For this review, use the dimensioned drawing (mm, ordinates from the lowest corner) and the shaded views. A direction names the side the tool comes from. Coordinates: 2 decimals unless noted, no trailing zeros. Loops run counter-clockwise (first coordinate to the right, second up) from the corner with the lowest first, then second, coordinate; pieces in that order, holes last. Notation, with made-up numbers: (56.5, 29) - (107.5, 29) arc R24 ccw to (107.5, 49) - close; hole circle Ø1 at (-22.75, 68.25). An arc over 180 degrees is marked (long way). Answer in a Markdown table with one row per item. Add a question column.
(1) For the marked faces 4, 5 and 6, list the 3-axis set-ups (+Z, -Z, +X, -X, +Y, -Y) from which the entire face can be reached by the end or side of a thin tool; tool diameter is ignored.
(2) The part is to be moulded in two halves that separate along Y. For the marked faces 1, 2 and 3, say which applies: released by +Y, released by -Y, zero draft, split by the parting line, or undercut.
(3) Clearance check with flat-ended pins moving along their axes: pin 1 (2 mm diameter, centred on x = 7.5, y = 4.5, fed in from +Z); pin 2 (1 mm diameter, centred on x = 19, z = 3, fed in from +Y). State where each tip first meets the part, or that it passes through.
(4) We need section B-B, the plane x = 11.25. Write out the cut boundary in (y, z), plus the area to 3 significant figures.
(5) To check wall thickness, follow L1, parallel to Y at x = 11, z = 4; L2, parallel to X at y = 9.5, z = 7.75; L3, parallel to Y at x = 16, z = 7.75. State the ranges of each line that lie inside material, in increasing order. Write a range as [from, to].
(6) We need section D-D, the plane y = 4.75. Write out the cut boundary in (x, z), plus the area to 3 significant figures.
(7) We need section C-C, the plane x = 17. Write out the cut boundary in (y, z), plus the area to 3 significant figures.
(8) We need section A-A, the plane y = 11.75. Write out the cut boundary in (x, z), plus the area to 3 significant figures.
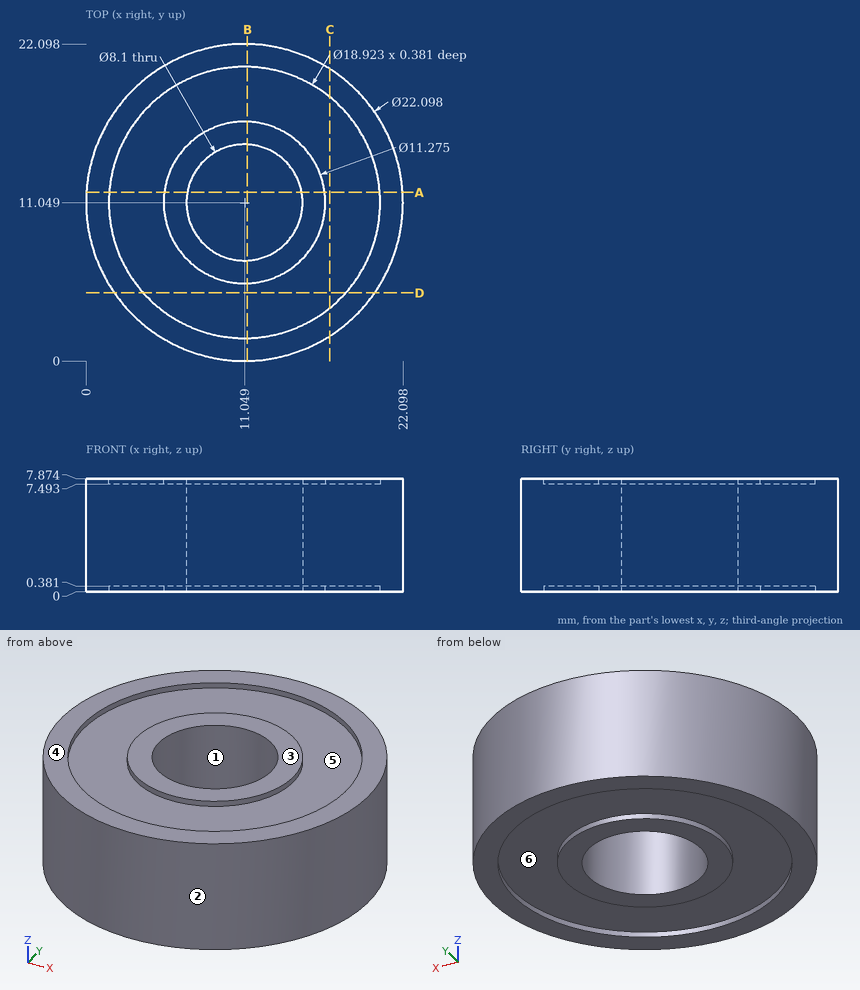
Responses:
| question | item | result |
|---|---|---|
| 1 | face 4 | +Z, +X, -X, +Y, -Y |
| 1 | face 5 | +Z |
| 1 | face 6 | -Z |
| 2 | face 1 | undercut |
| 2 | face 2 | split by the parting line |
| 2 | face 3 | zero draft |
| 3 | pin 1 | stops at z = 7.49 |
| 3 | pin 2 | stops at y = 19.21 |
| 4 | outline | (0, 0) - (1.59, 0) - (1.59, 0.38) - (5.42, 0.38) - (5.42, 0) - (7, 0) - (7, 7.87) - (5.42, 7.87) - (5.42, 7.49) - (1.59, 7.49) - (1.59, 7.87) - (0, 7.87) - close; (15.09, 0) - (16.68, 0) - (16.68, 0.38) - (20.51, 0.38) - (20.51, 0) - (22.1, 0) - (22.1, 7.87) - (20.51, 7.87) - (20.51, 7.49) - (16.68, 7.49) - (16.68, 7.87) - (15.09, 7.87) - close |
| 4 | area | 104 mm2 |
| 5 | L1 | y = [0, 7], [15.1, 22.1] |
| 5 | L2 | x = [0.11, 1.72], [5.63, 7.31], [14.79, 16.47], [20.38, 21.99] |
| 5 | L3 | y = [1.17, 2.99], [8.35, 13.75], [19.11, 20.93] |
| 6 | outline | (1.97, 0) - (3.99, 0) - (3.99, 0.38) - (18.11, 0.38) - (18.11, 0) - (20.13, 0) - (20.13, 7.87) - (18.11, 7.87) - (18.11, 7.49) - (3.99, 7.49) - (3.99, 7.87) - (1.97, 7.87) - close |
| 6 | area | 132 mm2 |
| 7 | outline | (1.74, 0) - (3.69, 0) - (3.69, 0.38) - (18.4, 0.38) - (18.4, 0) - (20.36, 0) - (20.36, 7.87) - (18.4, 7.87) - (18.4, 7.49) - (3.69, 7.49) - (3.69, 7.87) - (1.74, 7.87) - close |
| 7 | area | 135 mm2 |
| 8 | outline | (0.02, 0) - (1.61, 0) - (1.61, 0.38) - (5.46, 0.38) - (5.46, 0) - (7.06, 0) - (7.06, 7.87) - (5.46, 7.87) - (5.46, 7.49) - (1.61, 7.49) - (1.61, 7.87) - (0.02, 7.87) - close; (15.04, 0) - (16.64, 0) - (16.64, 0.38) - (20.48, 0.38) - (20.48, 0) - (22.08, 0) - (22.08, 7.87) - (20.48, 7.87) - (20.48, 7.49) - (16.64, 7.49) - (16.64, 7.87) - (15.04, 7.87) - close |
| 8 | area | 105 mm2 |
